Geometry: final body of the model. Coordinates: model frame, mm. A direction names the side the tool comes from. Give positions to 0.01 mm unless a question says otherwise; leave off trailing zeros. Write each loop counter-clockwise with the first axis right and the second up, starting at its lowest first coordinate (ties: lowest second). Pieces come first, ordered by that corner, then holes. Notation, with made-up numbers: M 9,85 L 21,85 A10 ccw 21,90 Z; hole C 64.5,88 d3. An arc over 180 degrees is marked long. Answer as a JSON object with one key per item and string values.
from build123d import *

# Parameters (mm, degrees)
SKETCH_R     = 10
PAD_DEPTH    = 1.5
SKETCH001_R  = 9.5
PAD001_DEPTH = 4
SKETCH002_R  = 10
PAD002_DEPTH = 1.5
SKETCH003_R  = 2.5
POCKET_DEPTH = 7.001


with BuildPart() as part:
    # Sketch → Pad (new body)
    with BuildSketch(Plane.XY):
        Circle(SKETCH_R)
    extrude(amount=PAD_DEPTH)

    # Sketch001 (on Face3 of Pad) → Pad001 (join)
    with BuildSketch(Plane.XY.offset(1.5)):
        Circle(SKETCH001_R)
    extrude(amount=PAD001_DEPTH)

    # Sketch002 (on Face5 of Pad001) → Pad002 (join)
    with BuildSketch(Plane.XY.offset(5.5)):
        Circle(SKETCH002_R)
    extrude(amount=PAD002_DEPTH)

    # Sketch003 (on Face3 of Pad002) → Pocket (cut, through all)
    with BuildSketch(Plane.XY.offset(7)):
        Circle(SKETCH003_R)
    extrude(amount=-POCKET_DEPTH, mode=Mode.SUBTRACT)


solid = part.part
1) Cut plane A-A on x = 0. Return loops of the section in (y, z), and give its area (3 significant figures).
Geometry check:
{"outline": "M -10,0 L -2.5,0 L -2.5,7 L -10,7 L -10,5.5 L -9.5,5.5 L -9.5,1.5 L -10,1.5 Z; M 2.5,0 L 10,0 L 10,1.5 L 9.5,1.5 L 9.5,5.5 L 10,5.5 L 10,7 L 2.5,7 Z", "area": "101 mm2"}
2) Contact query for a flat-ended pin moving along its axis: P1, Ø3, axis at y = -6.5, z = 4, coming from the +X side. Output: stop coordinate, or through.
Geometry check:
{"P1": "stops at x = 8.08"}
3) Cut plane D-D on x = 3. Return loops of the section in (y, z), and give its area (3 significant figures).
Geometry check:
{"outline": "M -9.54,0 L 9.54,0 L 9.54,1.5 L 9.01,1.5 L 9.01,5.5 L 9.54,5.5 L 9.54,7 L -9.54,7 L -9.54,5.5 L -9.01,5.5 L -9.01,1.5 L -9.54,1.5 Z", "area": "129 mm2"}
4) Set-up query: faces 1 (the flat face through (9, -4, 5.5)), 2 (the flat face through (2, -2, 0)). Return all of +Z, -Z, +X, -X, +Y, -Y with unobstructed straight access to the full face (end or side cutting, diameter ignored); none if empty.
Geometry check:
{"face 1": "none", "face 2": "-Z, +X, -X, +Y, -Y"}
5) Pull-direction query (Y, two-part tool) for faces 3 (the cylindrical face through (4.38, -8.43, 3.47)), 4 (the flat face through (9, -4, 1.5)), 5 (the cylindrical face through (-0.54, -2.44, 3.55)); classes: pulls with the +Y half, pulls with the -Y half, needs draft (parallel to the pull), parting line crosses it, or undercut.
Geometry check:
{"face 3": "parting line crosses it", "face 4": "needs draft", "face 5": "undercut"}
6) Line query: line 1 (Y direction, x = 0, z = 4.75); line 2 (X direction, y = -2, z = 4); line 3 (Y direction, x = -6, z = 3.75). Output: solid intervals per line, ascending. Write a range as from..to.
Geometry check:
{"line 1": "y = -9.5..-2.5, 2.5..9.5", "line 2": "x = -9.29..-1.5, 1.5..9.29", "line 3": "y = -7.37..7.37"}
7) Cut plane C-C on z = 3.25. Return loops of the section in (x, y), and give its area (3 significant figures).
Geometry check:
{"outline": "C 0,0 d19; hole C 0,0 d5", "area": "264 mm2"}
